The drawing under review shows one solid part. Ordinate dimensions are in mm from its lowest x, y, z. A direction names the side the tool comes from. Coordinates: 2 decimals unless noted, no trailing zeros. Order: outer loops, then holes, each group sorted by start corner. A loop starts at its lowest first (then second) coordinate and runs counter-clockwise, first axis right, second up. Notation, with made-up numbers: M 10,32 L 48,32 A9 cw 48,48 Z; hole C 68,40 d9. An arc over 180 degrees is marked long. Answer as a JSON object with one key per item and string values.
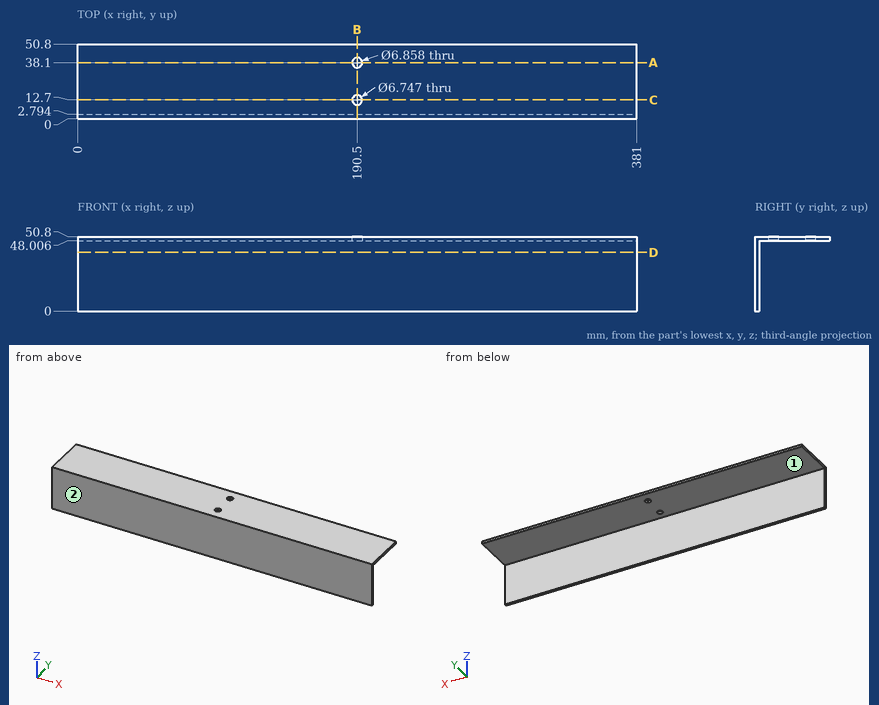
1) Add section D-D (z = 40). State the section outline as (x, y) points, and give its area (3 significant figures).
Taken from the geometry:
{"outline": "M 0,0 L 381,0 L 381,2.79 L 0,2.79 Z", "area": "1,060 mm2"}
2) Add section C-C (y = 12.7). State the section outline as (x, z) points.
Taken from the geometry:
{"outline": "M 0,48.01 L 187.13,48.01 L 187.13,50.8 L 0,50.8 Z; M 193.87,48.01 L 381,48.01 L 381,50.8 L 193.87,50.8 Z"}
3) To check wall thickness, follow L1, parallel to Y at x = 190.5, z = 50; L2, parallel to X at y = 12, z = 50; L3, parallel to X at y = 38, z = 49. State the ranges of each line that lie inside material, in increasing order.
Taken from the geometry:
{"L1": "y = 0 to 9.33, 16.07 to 34.67, 41.53 to 50.8", "L2": "x = 0 to 187.2, 193.8 to 381", "L3": "x = 0 to 187.07, 193.93 to 381"}
4) Insertion check: pin 1 Ø1 at (x, y) = (244, 6.5) entering from -Z; pin 2 Ø6 at (x, y) = (190.5, 12.7) entering from -Z; pin 3 Ø6 at (x, z) = (166.5, 39.5) entering from +Y. Each pin has a flat end and moves straight along its axis. Give the tip position at first contact, or say it passes through.
Taken from the geometry:
{"pin 1": "stops at z = 48.01", "pin 2": "passes through", "pin 3": "stops at y = 2.79"}
5) Add section B-B (x = 190.5). State the section outline as (y, z) points, and give its area (3 significant figures).
Taken from the geometry:
{"outline": "M 0,0 L 2.79,0 L 2.79,48.01 L 9.33,48.01 L 9.33,50.8 L 0,50.8 Z; M 16.07,48.01 L 34.67,48.01 L 34.67,50.8 L 16.07,50.8 Z; M 41.53,48.01 L 50.8,48.01 L 50.8,50.8 L 41.53,50.8 Z", "area": "238 mm2"}
6) Add section A-A (y = 38.1). State the section outline as (x, z) points.
Taken from the geometry:
{"outline": "M 0,48.01 L 187.07,48.01 L 187.07,50.8 L 0,50.8 Z; M 193.93,48.01 L 381,48.01 L 381,50.8 L 193.93,50.8 Z"}
7) Tool access review of the marked faces 1 and 2: name each direction out of +Z, -Z, +X, -X, +Y, -Y from which nothing blocks a thin tool from reaching the whole face with its end or side.
Taken from the geometry:
{"face 1": "-Z, +X, -X, +Y", "face 2": "+Z, -Z, +X, -X, -Y"}
